Autodesk Inventor part; units mm, degrees
ref_plane "YZ Plane" through (0, 0, 0) normal (1, 0, 0) x (0, 1, 0)
ref_plane "XZ Plane" through (0, 0, 0) normal (0, 1, 0) x (-1, 0, 0)
ref_plane "XY Plane" through (0, 0, 0) normal (0, 0, 1) x (1, 0, 0)
sketch "Sketch1" plane through (0, 0, 0) normal (0, 0, 1) x (1, 0, 0)
  line L0 (0, 0) -> (24, 0)
  line L1 (24, 0) -> (24, -60)
  line L2 (24, -60) -> (0, -60)
  line L3 (0, -60) -> (0, 0)
  dimension "d0" = 24
  dimension "d1" = 60
extrude "Extrusion1" add sketch "Sketch1" along normal blind 2
sketch "Sketch2" plane through (0, 0, 2) normal (0, 0, 1) x (1, 0, 0)
  line L0 (0, -60) -> (24, -60)
  line L1 (0, 0) -> (2, 0)
  line L2 (2, 0) -> (2, -60)
  line L3 (2, -60) -> (0, -60)
  line L4 (0, -60) -> (0, 0)
  line L5 (24, -60) -> (24, 0)
  line L6 (24, 0) -> (22, 0)
  line L7 (22, 0) -> (22, -60)
  line L8 (22, -60) -> (24, -60)
  line L9 (24, -60) -> (24, 0)
  dimension "d4" = 2
  dimension "d5" = 2
extrude "Extrusion2" add sketch "Sketch2" along normal blind 15
sketch "Sketch3" plane through (24, -60, 0) normal (1, 0, 0) x (0, 0, -1)
  circle A0 centre (-8.5, 57) radius 1
  circle A1 centre (-8.5, 29.5) radius 1
  line L0 (-17, 0) -> (-17, 60)
  line L1 (0, 60) -> (-17, 60)
  dimension "d8" = 2
  dimension "d9" = 2
  dimension "d10" = 8.5
  dimension "d11" = 8.5
  dimension "d12" = 27.5
  dimension "d13" = 3
extrude "Extrusion3" cut sketch "Sketch3" against normal up to surface (2 mm away)
sketch "Sketch4" plane through (24, -60, 0) normal (1, 0, 0) x (0, 0, -1)
  line L0 (-17, 60) -> (-17, 0)
  line L1 (-17, 55) -> (-2, 55)
  line L2 (-2, 55) -> (-2, 31.5)
  line L3 (-2, 31.5) -> (-17, 31.5)
  line L4 (-17, 31.5) -> (-17, 55)
  circle A0 centre (-8.5, 57) radius 1
  circle A1 centre (-8.5, 29.5) radius 1
  point P0 (-17, 31.5)
  dimension "d23" = 15
  dimension "d24" = 23.5
  dimension "d25" = 2
  dimension "d26" = 2
extrude "Extrusion4" cut sketch "Sketch4" against normal up to surface (2 mm away) contours L1 L2 L3 L0
sketch "Sketch5" plane through (0, -60, 0) normal (-1, 0, 0) x (0, 0, 1)
  circle A0 centre (8.5, 48.4) radius 2.5
  circle A1 centre (8.5, 57) radius 1
  point P0 (0, 60)
  dimension "d29" = 5
  dimension "d32" = 8.6
  dimension "d33" = 0
extrude "Extrusion5" add sketch "Sketch5" along normal blind 5 contours A0
sketch "Sketch12" plane through (0, 0, 0) normal (0, 0, -1) x (-1, 0, 0)
  line L0 (3, -60) -> (-35, -60)
  line L1 (-35, -60) -> (-35, -85)
  line L2 (-35, -85) -> (3, -85)
  line L3 (3, -85) -> (3, -60)
  line L4 (0, 0) -> (0, -60)
  line L5 (-2, -60) -> (-22, -60)
  line L6 (3, -60) -> (0, -60)
  line L7 (0, -60) -> (0, -85)
  line L8 (0, -85) -> (3, -85)
  line L9 (3, -85) -> (3, -60)
  line L10 (-35, -60) -> (-30, -60)
  line L11 (-30, -60) -> (-30, -85)
  line L12 (-30, -85) -> (-35, -85)
  line L13 (-35, -85) -> (-35, -60)
  line L14 (-30, -60) -> (-32, -60)
  line L15 (-32, -60) -> (-32, -75)
  line L16 (-32, -75) -> (-30, -75)
  line L17 (-30, -75) -> (-30, -60)
  dimension "d51" = 38
  dimension "d52" = 3
  dimension "d53" = 25
  dimension "d54" = 0
  dimension "d55" = 3
  dimension "d56" = 5
  dimension "d95" = 2
  dimension "d96" = 15
extrude "Extrusion9" add sketch "Sketch12" against normal up to surface (17 mm away) contours L3 L2 L7 L0 | L2 L1 L0 L15 L16 L11
sketch "Sketch13" plane through (0, 0, 0) normal (0, 0, -1) x (-1, 0, 0)
  line L0 (-32, -60) -> (-35, -60)
  line L1 (0, -60) -> (-24, -60)
  line L2 (-35, -60) -> (-24, -60)
  line L3 (-24, -60) -> (-24, -45)
  line L4 (-24, -45) -> (-35, -60)
  line L5 (0, -60) -> (0, -45)
  line L6 (0, 0) -> (0, -60)
  line L7 (0, -60) -> (15, -60) construction
  line L8 (0, -45) -> (3, -60)
  line L9 (3, -60) -> (0, -60)
  point P0 (-30, -60)
  dimension "d59" = 15
  dimension "d60" = 90
  dimension "d63" = 15
  dimension "d64" = 90
extrude "Extrusion10" add sketch "Sketch13" against normal up to surface (17 mm away)
sketch "Sketch14" plane through (-3, -85, 0) normal (-1, 0, 0) x (0, 0, 1)
  circle A0 centre (8.5, 5) radius 2.5
  line L0 (17, 0) -> (17, 25)
  line L1 (0, 25) -> (17, 25)
  point P0 (0, 85)
  dimension "d65" = 5
  dimension "d66" = 8.5
  dimension "d67" = 20
extrude "Extrusion11" cut sketch "Sketch14" against normal up to surface (38 mm away)
sketch "Sketch15" plane through (2, -60, 2) normal (1, 0, 0) x (0, 0, -1)
  line L0 (2, 0) -> (-15, 0)
  line L1 (-15, 60) -> (-13, 60)
  line L2 (-13, 60) -> (-13, 0)
  line L3 (-13, 0) -> (-15, 0)
  line L4 (-15, 0) -> (-15, 60)
  point P0 (2, 60)
  dimension "d70" = 2
extrude "Extrusion12" add sketch "Sketch15" along normal up to surface (22 mm away)
sketch "Sketch16" plane through (0, 0, 0) normal (0, 0, -1) x (-1, 0, 0)
  line L0 (-2, 0) -> (-2, -60)
  line L1 (-2, -60) -> (-22, -60)
  line L2 (-2, 0) -> (-22, 0)
  line L3 (-22, 0) -> (-22, -60)
  line L4 (-22, -60) -> (-2, -60)
  line L5 (-2, -60) -> (-2, 0)
  line L6 (-24, -45) -> (-24, 0)
  line L7 (-24, -28.5) -> (-22, -28.5)
  line L8 (-24, -5) -> (-22, -5)
  line L9 (-22, -5) -> (-22, -28.5)
  line L10 (-22, -28.5) -> (-24, -28.5)
  line L11 (-24, -28.5) -> (-24, -5)
  point P0 (0, 0)
extrude "Extrusion14" cut sketch "Sketch16" against normal up to surface (2 mm away)
sketch "Sketch17" plane through (22, -60, 0) normal (0, -1, 0) x (1, 0, 0)
  line L0 (-20, 2) -> (-20, 15)
  line L1 (-20, 15) -> (0, 15)
  line L2 (-20, 0) -> (0, 0)
  line L3 (0, 0) -> (0, 15)
  line L4 (0, 15) -> (-20, 15)
  line L5 (-20, 15) -> (-20, 0)
  point P0 (-22, 0)
  point P1 (-20, 2)
extrude "Extrusion15" add sketch "Sketch17" against normal blind 2
sketch "Sketch18" plane through (0, 0, 0) normal (0, 1, 0) x (1, 0, 0)
  line L0 (0, 0) -> (0, -17)
  line L1 (24, -17) -> (24, 0)
  line L2 (0, -17) -> (24, -17)
  line L3 (24, -17) -> (24, 0)
  line L4 (24, 0) -> (0, 0)
  line L5 (0, 0) -> (0, -17)
extrude "Extrusion16" add sketch "Sketch18" along normal blind 2
sketch "Sketch19" plane through (0, 2, 0) normal (0, 1, 0) x (1, 0, 0)
  circle A0 centre (12, -8.5) radius 6
  line L0 (0, 0) -> (0, -17)
  line L1 (0, -17) -> (24, -17)
  dimension "d81" = 12
  dimension "d82" = 12
  dimension "d83" = 8.5
extrude "Extrusion17" cut sketch "Sketch19" against normal up to surface (62 mm away)
sketch "Sketch20" plane through (35, -85, 17) normal (1, 0, 0) x (0, 0, -1)
  circle A0 centre (8.5, 5) radius 2.5
  circle A1 centre (8.5, 5) radius 3.75
  point P0 (17, 85)
  dimension "d86" = 7.5
extrude "Extrusion18" cut sketch "Sketch20" against normal up to surface (5 mm away)
fillet "Fillet2" radius 8.5 4 edges at (-1.5, -85, 0) (-1.5, -85, 17) (32.5, -85, 0) (32.5, -85, 17)
sketch "Sketch21" plane through (35, -60, 17) normal (1, 0, 0) x (0, 0, -1)
  circle A0 centre (8.5, -20) radius 3.75
  circle A1 centre (8.5, -20) radius 3.75
  circle A2 centre (8.5, -5) radius 2
  circle A3 centre (8.5, -20) radius 3.75
  line L0 (10.4863, -4.7667) -> (12.2244, -19.5625)
  line L1 (6.5137, -4.7667) -> (4.7756, -19.5625)
  point P0 (17, 60)
  point P1 (4.7756, -19.5625)
  point P2 (12.2244, -19.5625)
  dimension "d90" = 4
  dimension "d91" = 15
  dimension "d92" = 0
extrude "Extrusion19" cut sketch "Sketch21" against normal blind 3
properties part number "juncao5"
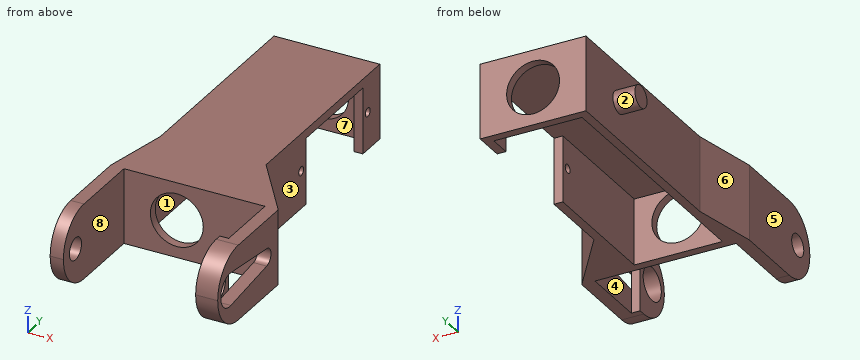
Build history of the part. All positions in model axes, mm. Face numbers are marked on the shaded views. A direction names the side the tool comes from. Coordinates: 2 decimals unless noted, no trailing zeros. Order: outer loops, then holes, each group sorted by start corner. A loop starts at its lowest first (then second) coordinate and runs counter-clockwise, first axis right, second up. Notation, with made-up numbers: (-15.5, 52) -> (23.5, 52) arc R33 cw to (23.5, 85) -> close; hole circle Ø8 at (30, -9.5). An arc over 180 degrees is marked (long way). Answer in a Markdown table with one row per item. Add a question column.
Q1. Wall check: line 1 along Y through (x, z) = (23.4, 8.5); line 2 along Y through (x, z) = (3, 4.5); line 3 along Y through (x, z) = (23.5, 6). Give the ranges that are in metal, low to high. Write a range as [from, to].
Q2. Mould opens along X. For the marked faces 1, 2 and 3 say: +X half, -X half, draft (parallel to the pull), parting line (faces both ways), or undercut.
Q3. Which spindle directions (+Z, -Z, +X, -X, +Y, -Y) get a long thin tool onto all of the face, cutting with end or side? Do the marked faces 4, 5, 6, 7 and 8. Say none if no direction does.
Q4. Band-saw the part on C-C, the plane y = -74. List the corners of the cut face in (x, z), then the cut area to 3 significant figures.
Q5. Band-saw the part on B-B, the plane x = 5. List the corners of the cut face in (y, z).
Q6. Band-saw the part on A-A, the plane y = -3. List the corners of the cut face in (x, z).
Q7. Band-saw the part on D-D, the plane x = 17. List the corners of the cut face in (y, z), then the cut area to 3 significant figures.
Q8. Drop flat-ended pins along their axis: pin 1 (6 mm diameter, centred on x = 7, z = 10.5, fed in from -Y); pin 2 (5.5 mm diameter, centred on y = -2, z = 6.5, fed in from -X); pin 3 (7.5 mm diameter, centred on x = 13, z = 9.5, fed in from -Y); pin 4 (7.5 mm diameter, centred on y = -64, z = 8.5, fed in from -X). Give the stop position or say it passes through.
Answers follow:
| question | item | result |
|---|---|---|
| 1 | line 1 | [-60, -31.5], [-29.5, -28.5], [-5, -4], [-2, 2] |
| 1 | line 2 | [-60, -58], [0, 2] |
| 1 | line 3 | [-60, -28.5], [-5, 2] |
| 2 | face 1 | undercut |
| 2 | face 2 | draft |
| 2 | face 3 | +X half |
| 3 | face 4 | +Z, -Z |
| 3 | face 5 | +Z, -Z, -X, -Y |
| 3 | face 6 | +Z, -Z, -X |
| 3 | face 7 | -Z |
| 3 | face 8 | +Z, -Z, -Y |
| 4 | outline | (-3, 0) -> (0, 0) -> (0, 17) -> (-3, 17) -> close; (32, 0) -> (35, 0) -> (35, 5.43) -> (32, 5.43) -> close; (32, 11.57) -> (35, 11.57) -> (35, 17) -> (32, 17) -> close |
| 4 | area | 83.6 mm^2 |
| 5 | outline | (-60, 0) -> (-58, 0) -> (-58, 15) -> (0, 15) -> (0, 0) -> (2, 0) -> (2, 17) -> (-60, 17) -> close |
| 6 | outline | (0, 0) -> (2, 0) -> (2, 15) -> (22, 15) -> (22, 9.5) -> (24, 9.5) -> (24, 17) -> (0, 17) -> close; (22, 0) -> (24, 0) -> (24, 7.5) -> (22, 7.5) -> close |
| 7 | outline | (-60, 0) -> (-58, 0) -> (-58, 5.18) -> (-60, 5.18) -> close; (-60, 11.82) -> (-58, 11.82) -> (-58, 15) -> (0, 15) -> (0, 11.82) -> (2, 11.82) -> (2, 17) -> (-60, 17) -> close; (0, 0) -> (2, 0) -> (2, 5.18) -> (0, 5.18) -> close |
| 7 | area | 157 mm^2 |
| 8 | pin 1 | y = -60 |
| 8 | pin 2 | x = 0 |
| 8 | pin 3 | through |
| 8 | pin 4 | x = -3 |
